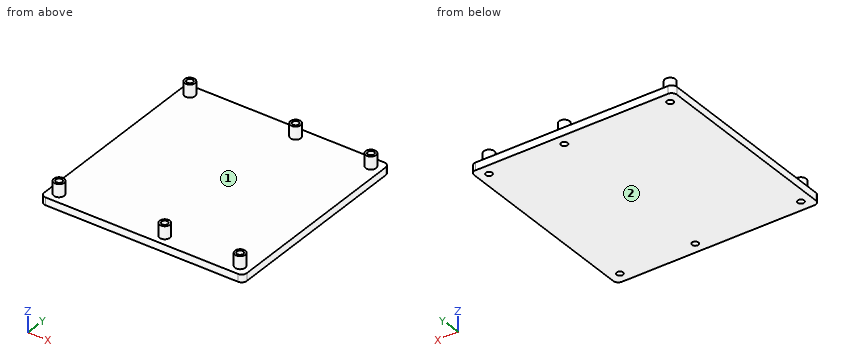
from build123d import *

# Parameters (mm, degrees)
F3_DEPTH = 3
F1_R     = 2.05
F4_DEPTH = 8
F2_R     = 1.25
F5_DEPTH = 8.001


with BuildPart() as f3:
    # F0 (on Top) → F3 (new body)
    with BuildSketch(Plane.XY):
        with BuildLine():
            Line((38, 40), (-38, 40))
            ThreePointArc((-38, 40), (-39.414214, 39.414214), (-40, 38))
            Line((-40, 38), (-40, -38))
            ThreePointArc((-40, -38), (-39.414214, -39.414214), (-38, -40))
            Line((-38, -40), (38, -40))
            ThreePointArc((38, -40), (39.414214, -39.414214), (40, -38))
            Line((40, -38), (40, 38))
            ThreePointArc((40, 38), (39.414214, 39.414214), (38, 40))
        make_face()
    extrude(amount=F3_DEPTH)

    # F1 (on Top) → F4 (join)
    with BuildSketch(Plane.XY):
        with Locations((-35.75, 35.75)):
            Circle(F1_R)
        with Locations((6, 35.75)):
            Circle(F1_R)
        with Locations((35.75, 35.75)):
            Circle(F1_R)
        with Locations((35.75, -35.75)):
            Circle(F1_R)
        with Locations((6, -35.75)):
            Circle(F1_R)
        with Locations((-35.75, -35.75)):
            Circle(F1_R)
    extrude(amount=F4_DEPTH)

    # F2 (on Top) → F5 (cut, through all)
    with BuildSketch(Plane.XY):
        with Locations((-35.75, 35.75)):
            Circle(F2_R)
        with Locations((6, 35.75)):
            Circle(F2_R)
        with Locations((35.75, 35.75)):
            Circle(F2_R)
        with Locations((35.75, -35.75)):
            Circle(F2_R)
        with Locations((6, -35.75)):
            Circle(F2_R)
        with Locations((-35.75, -35.75)):
            Circle(F2_R)
    extrude(amount=F5_DEPTH, mode=Mode.SUBTRACT)


solid = f3.part
Model file for the job. Use its own axes, mm. Face numbers are marked on the shaded views. A direction names the side the tool comes from. Give positions to 0.01 mm unless a question says otherwise; leave off trailing zeros. Write each loop counter-clockwise with the first axis right and the second up, starting at its lowest first coordinate (ties: lowest second). Pieces come first, ordered by that corner, then holes. Notation, with made-up numbers: (-3.5, 28) -> (24.5, 28) arc R27 cw to (24.5, 63) -> close; hole circle Ø7 at (65, 85). An arc over 180 degrees is marked (long way). Write item = value, one per line.
(1) Slice it at D-D, the plane x = -30.5. Give the cut face in (y, z), then the cut area to 3 significant figures.
Determined:
outline = (-40, 0) -> (40, 0) -> (40, 3) -> (-40, 3) -> close
area = 240 mm2
(2) Probe line 1 along X through (y, z) = (-35.75, 2.5); line 2 along X through (y, z) = (35.75, 3.5); line 3 along Y through (x, z) = (-35.75, 3.75). List the from-to ranges inside material, lowest first.
Determined:
line_1 = -40 to -37, -34.5 to 4.75, 7.25 to 34.5, 37 to 40
line_2 = -37.8 to -37, -34.5 to -33.7, 3.95 to 4.75, 7.25 to 8.05, 33.7 to 34.5, 37 to 37.8
line_3 = -37.8 to -37, -34.5 to -33.7, 33.7 to 34.5, 37 to 37.8
(3) Slice it at C-C, the plane x = 35.75. Give the cut face in (y, z), then the cut area to 3 significant figures.
Determined:
outline = (-40, 0) -> (-37, 0) -> (-37, 8) -> (-37.8, 8) -> (-37.8, 3) -> (-40, 3) -> close; (-34.5, 0) -> (34.5, 0) -> (34.5, 8) -> (33.7, 8) -> (33.7, 3) -> (-33.7, 3) -> (-33.7, 8) -> (-34.5, 8) -> close; (37, 0) -> (40, 0) -> (40, 3) -> (37.8, 3) -> (37.8, 8) -> (37, 8) -> close
area = 241 mm2
(4) Tool access for the marked faces 1 and 2: list every direction of +Z, -Z, +X, -X, +Y, -Y with a clear straight run to the whole face (end or side of a thin tool).
Determined:
face_1 = +Z
face_2 = -Z, +X, -X, +Y, -Y
(5) Slice it at A-A, the plane z = 6. Give the number of separate pieces and of enclosed holes in the cut face, then the cut area to 3 significant figures.
Determined:
separate_pieces = 6
enclosed_holes = 6
area = 49.8 mm2
(6) Slice it at B-B, the plane y = -35.75. Give the cut face in (x, z), then the cut area to 4 significant figures.
Determined:
outline = (-40, 0) -> (-37, 0) -> (-37, 8) -> (-37.8, 8) -> (-37.8, 3) -> (-40, 3) -> close; (-34.5, 0) -> (4.75, 0) -> (4.75, 8) -> (3.95, 8) -> (3.95, 3) -> (-33.7, 3) -> (-33.7, 8) -> (-34.5, 8) -> close; (7.25, 0) -> (34.5, 0) -> (34.5, 8) -> (33.7, 8) -> (33.7, 3) -> (8.05, 3) -> (8.05, 8) -> (7.25, 8) -> close; (37, 0) -> (40, 0) -> (40, 3) -> (37.8, 3) -> (37.8, 8) -> (37, 8) -> close
area = 241.5 mm2
(7) Flat gauge pins, fed straight in: P1, Ø3, axis at x = 10.5, z = 5, coming from the +Y side; P2, Ø1, axis at x = 12, y = 27.5, coming from the +Z side. Where does each tip first touch, or does it go through?
Determined:
P1 = through
P2 = 3
